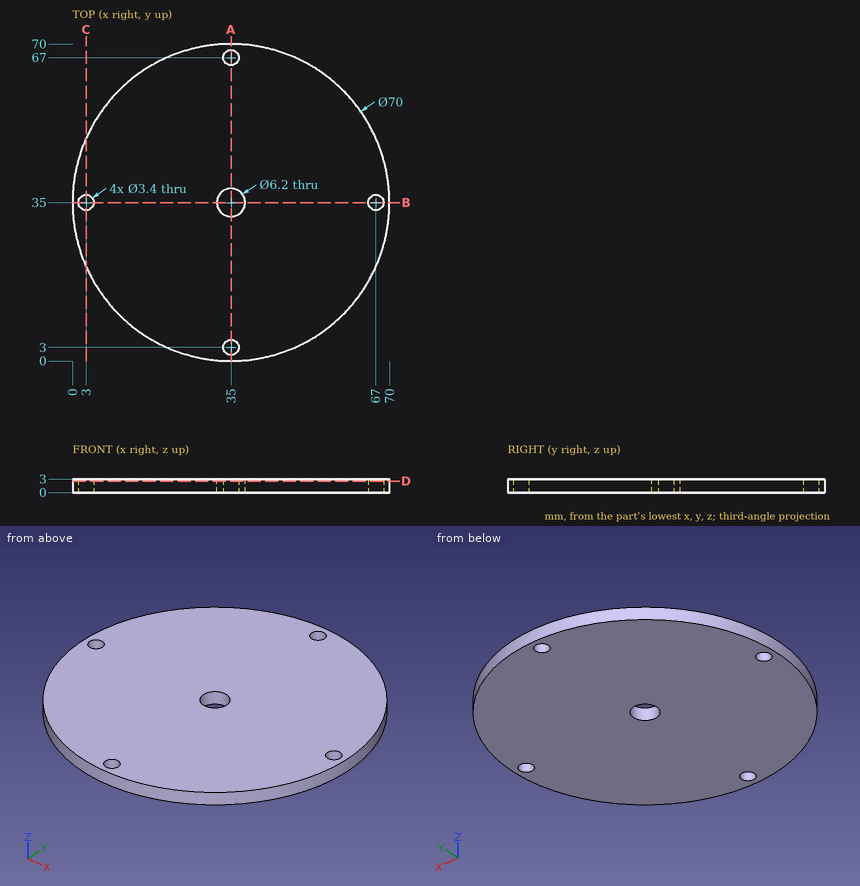
Print and shaded views of the part. All mm, measured from the part's lowest x, y and z. Give positions to 0.01 mm unless a question says otherwise; leave off trailing zeros. Order: outer loops, then holes, each group sorted by start corner. A loop starts at its lowest first (then second) coordinate and runs counter-clockwise, first axis right, second up. Notation, with made-up numbers: (32, 51.25) - (54, 51.25) arc R22 cw to (54, 86.25) - close; hole circle Ø4 at (41.5, 17). An arc over 180 degrees is marked (long way). Use a Markdown table: item, result.
1) Saw through at A-A on x = 35. List the corners of the cut face in (y, z).
Checked values:
| item | result |
|---|---|
| outline | (0, 0) - (1.3, 0) - (1.3, 3) - (0, 3) - close; (4.7, 0) - (31.9, 0) - (31.9, 3) - (4.7, 3) - close; (38.1, 0) - (65.3, 0) - (65.3, 3) - (38.1, 3) - close; (68.7, 0) - (70, 0) - (70, 3) - (68.7, 3) - close |
2) Probe L1, parallel to Y at x = 35, z = 2.1; L2, parallel to Y at x = 67, z = 1.05; L3, parallel to X at y = 37, z = 2.4. List the from-to ranges inside material, lowest first. Write a range as from..to.
Checked values:
| item | result |
|---|---|
| L1 | 0..1.3, 4.7..31.9, 38.1..65.3, 68.7..70 |
| L2 | 20.82..33.3, 36.7..49.18 |
| L3 | 0.06..32.63, 37.37..69.94 |
3) Flat gauge pins, fed straight in: P1, Ø1.5, axis at x = 52, z = 1.5, coming from the -Y side; P2, Ø2.5, axis at x = 3, y = 35, coming from the -Z side; P3, Ø1.5, axis at y = 27.5, z = 1, coming from the +X side; P4, Ø1.5, axis at x = 9.5, z = 1, coming from the +Y side. Where does each tip first touch, or does it go through?
Checked values:
| item | result |
|---|---|
| P1 | y = 4 |
| P2 | through |
| P3 | x = 69.34 |
| P4 | y = 59.75 |
4) Saw through at C-C on x = 3. List the corners of the cut face in (y, z).
Checked values:
| item | result |
|---|---|
| outline | (20.82, 0) - (33.3, 0) - (33.3, 3) - (20.82, 3) - close; (36.7, 0) - (49.18, 0) - (49.18, 3) - (36.7, 3) - close |
5) Saw through at D-D on z = 2.55. List the corners of the cut face in (x, y), plus the area to 3 significant figures.
Checked values:
| item | result |
|---|---|
| outline | circle Ø70 at (35, 35); hole circle Ø3.4 at (3, 35); hole circle Ø6.2 at (35, 35); hole circle Ø3.4 at (35, 3); hole circle Ø3.4 at (35, 67); hole circle Ø3.4 at (67, 35) |
| area | 3,780 mm² |
